Design review of the part built by this model. Coordinates are the model's own, in mm. Face numbers are marked on the shaded views. Coordinates: 2 decimals unless noted, no trailing zeros. Write each loop counter-clockwise with the first axis right and the second up, starting at its lowest first coordinate (ties: lowest second). Pieces come first, ordered by that corner, then holes. Notation, with made-up numbers: M 12,-23 L 34,-23 A26 cw 34,8 Z; hole C 15.25,57 d10. An arc over 180 degrees is marked long. Return JSON: item names as keys, results as strings. Group by question number.
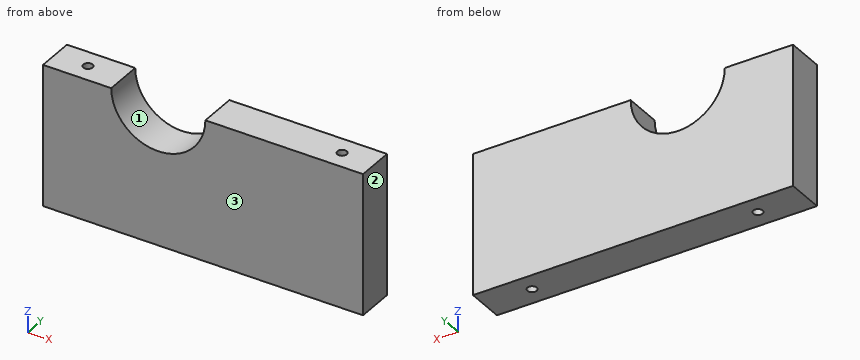
```python
from build123d import *

# Parameters (mm, degrees)
BOSS_EXTRUDE1_DEPTH = 8
CUT_EXTRUDE5_START  = 4
SKETCH2_R           = 1
CUT_EXTRUDE5_DEPTH  = 5
CUT_EXTRUDE6_START  = -27.204301
SKETCH3_R           = 1
CUT_EXTRUDE6_DEPTH  = 10


with BuildPart() as part:
    # Sketch1 → Boss-Extrude1 (new body)
    with BuildSketch(Plane(origin=(0, 0, 0), x_dir=(1, 0, 0), z_dir=(0, 1, 0))):
        with BuildLine():
            Line((-40.967741935, 27.204301075), (27.032258065, 27.204301075))
            Line((27.032258065, 27.204301075), (27.032258065, -2.795698925))
            Line((27.032258065, -2.795698925), (-6.467741935, -2.795698925))
            ThreePointArc((-6.467741935, -2.795698925), (-16.467741935, 7.204301075), (-26.467741935, -2.795698925))
            Line((-26.467741935, -2.795698925), (-40.967741935, -2.795698925))
            Line((-40.967741935, -2.795698925), (-40.967741935, 27.204301075))
        make_face()
    extrude(amount=BOSS_EXTRUDE1_DEPTH)

    # Sketch2 → Cut-Extrude5 (cut)
    with BuildSketch(Plane.XY.offset(CUT_EXTRUDE5_START)):
        with Locations((-33.967741935, 4)):
            Circle(SKETCH2_R)
        with Locations((20.032258065, 4)):
            Circle(SKETCH2_R)
    extrude(amount=-CUT_EXTRUDE5_DEPTH, mode=Mode.SUBTRACT)

    # Sketch3 → Cut-Extrude6 (cut)
    with BuildSketch(Plane.XY.offset(CUT_EXTRUDE6_START)):
        with Locations((17.032258065, 4)):
            Circle(SKETCH3_R)
        with Locations((-30.967741935, 4)):
            Circle(SKETCH3_R)
    extrude(amount=CUT_EXTRUDE6_DEPTH, mode=Mode.SUBTRACT)


solid = part.part
```
Item 1: Add section B-B (y = 2). Write out the cut boundary in (x, z).
Item 2: For pin 1 (2.5 mm diameter, centred on x = 17.03, y = 4, fed in from -Z); pin 2 (0.6 mm diameter, centred on x = 20, y = 4, fed in from +Z); pin 3 (6 mm diameter, centred on x = -16, z = -2, fed in from -Y), all flat-tipped, find the tip position at first contact; note any pin that passes through.
Item 3: Add section A-A (z = -4.75). Write out the cut boundary in (x, y), plus the area to 3 significant figures.
Item 4: Add section C-C (x = -9.5). Write out the cut boundary in (y, z), plus the area to 3 significant figures.
Item 5: The part is to be moulded in two halves that separate along X. For the marked faces 1, 2 and 3, say which applies: pulls with the +X half, pulls with the -X half, needs draft (parallel to the pull), parting line crosses it, or undercut.
Item 6: For line 1 (X direction, y = 1.5, z = -2.5); line 2 (Z direction, x = -17, y = 1); line 3 (X direction, y = 7, z = -6), list the stretches that pass through material, from the lowest coordinate up.
Geometry check:
{
 "1": {"outline": "M -40.97,-27.2 L 27.03,-27.2 L 27.03,2.8 L -6.47,2.8 A10 cw -26.47,2.8 L -40.97,2.8 Z"},
 "2": {"pin 1": "z = -27.2", "pin 2": "z = -1", "pin 3": "through"},
 "3": {"outline": "M -40.97,0 L -23.03,0 L -23.03,8 L -40.97,8 Z; M -9.91,0 L 27.03,0 L 27.03,8 L -9.91,8 Z", "area": "439 mm^2"},
 "4": {"outline": "M 0,-27.2 L 8,-27.2 L 8,-4.38 L 0,-4.38 Z", "area": "183 mm^2"},
 "5": {"face 1": "undercut", "face 2": "pulls with the +X half", "face 3": "needs draft"},
 "6": {"line 1": "-40.97 to -24.95, -7.99 to 27.03", "line 2": "-27.2 to -7.19", "line 3": "-40.97 to -21.23, -11.71 to 27.03"}
}
